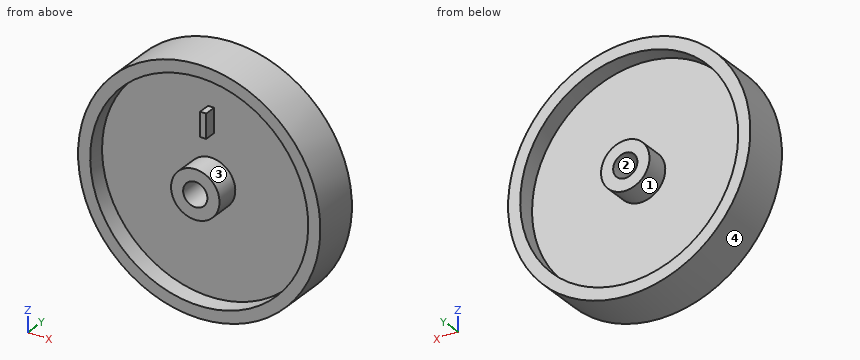
from build123d import *

# Parameters (mm, degrees)
F3_W     = 2.5
F3_H     = 10
F4_DEPTH = 5


with BuildPart() as f2:
    # F0 (on Right) → F2 (revolve)
    with BuildSketch(Plane.YZ):
        Polygon((-25, 5), (0, 5), (0, 10), (-10, 10), (-10, 45), (-2.5, 45), (-2.5, 50), (-22.5, 50), (-22.5, 45), (-15, 45), (-15, 10), (-25, 10), align=None)
    revolve(axis=Axis((0, -23.925491, 0), (0, -1, 0)))

    # F3 (on face) → F4 (join)
    with BuildSketch(Plane.XZ.offset(15)):
        with Locations((0, 25)):
            Rectangle(F3_W, F3_H)
    extrude(amount=F4_DEPTH)


solid = f2.part
Read the model definition and answer for the solid it produces. Units are mm, in the model's axes. Face numbers are marked on the shaded views. A direction names the side the tool comes from. Coordinates: 2 decimals unless noted, no trailing zeros. Write each loop counter-clockwise with the first axis right and the second up, starting at its lowest first coordinate (ties: lowest second). Pieces come first, ordered by that corner, then holes. Notation, with made-up numbers: (-34.5, 22) - (12.5, 22) arc R25 cw to (12.5, 59) - close; hole circle Ø4 at (74.25, 66.5). An arc over 180 degrees is marked (long way). One line per question, with ' | ' between items.
Q1. Find section B-B, the plane x = 0. Write down the section's boundary in (y, z), plus the area to 3 significant figures.
Result set:
outline: (-25, -10) - (-15, -10) - (-15, -45) - (-22.5, -45) - (-22.5, -50) - (-2.5, -50) - (-2.5, -45) - (-10, -45) - (-10, -10) - (0, -10) - (0, -5) - (-25, -5) - close; (-25, 5) - (0, 5) - (0, 10) - (-10, 10) - (-10, 45) - (-2.5, 45) - (-2.5, 50) - (-22.5, 50) - (-22.5, 45) - (-15, 45) - (-15, 30) - (-20, 30) - (-20, 20) - (-15, 20) - (-15, 10) - (-25, 10) - close | area: 850 mm^2
Q2. For the marked faces 1 and 2, determine the directions among +Z, -Z, +X, -X, +Y, -Y from which every point of the face is accessible in a straight line to the end or side of a thin tool.
Result set:
face 1: +Y | face 2: +Y, -Y
Q3. Determine the mould class of the marked faces 3 and 4 for opening direction Z: +Z half, -Z half, draft (parallel to the pull), parting line (faces both ways), or undercut.
Result set:
face 3: undercut | face 4: parting line
Q4. Each of these flat-tipped pins is pushed along its axis until it touches: P1, Ø2.5, axis at y = -18, z = 23.5, coming from the -X side; P2, Ø4, axis at x = 33.5, z = -14.5, coming from the +Y side; P3, Ø2.5, axis at y = -17.5, z = 27, coming from the +X side. Where does it stop, or does it pass through?
Result set:
P1: x = -44.78 | P2: y = -10 | P3: x = 42.86
Q5. Find section C-C, the plane z = 0. Write down the section's boundary in (x, y), plus the area to 3 significant figures.
Result set:
outline: (-50, -22.5) - (-45, -22.5) - (-45, -15) - (-10, -15) - (-10, -25) - (-5, -25) - (-5, 0) - (-10, 0) - (-10, -10) - (-45, -10) - (-45, -2.5) - (-50, -2.5) - close; (5, -25) - (10, -25) - (10, -15) - (45, -15) - (45, -22.5) - (50, -22.5) - (50, -2.5) - (45, -2.5) - (45, -10) - (10, -10) - (10, 0) - (5, 0) - close | area: 800 mm^2
Q6. Consider L1, parallel to Z at x = 0, y = -19; L2, parallel to Z at x = 0, y = -20.25. Determine where each line is inside the solid, lowest interval first. Write a range as [from, to].
Result set:
L1: [-50, -45], [-10, -5], [5, 10], [20, 30], [45, 50] | L2: [-50, -45], [-10, -5], [5, 10], [45, 50]
Q7. Find section A-A, the plane y = -18.5. Write down the section's boundary in (x, z).
Result set:
outline: circle Ø100 at (0, 0); circle Ø20 at (0, 0); (-1.25, 20) - (1.25, 20) - (1.25, 30) - (-1.25, 30) - close; hole circle Ø90 at (0, 0); hole circle Ø10 at (0, 0)
Q8. Find section D-D, the plane z = 23. Write down the section's boundary in (x, y).
Result set:
outline: (-44.4, -22.5) - (-38.68, -22.5) - (-38.68, -15) - (-1.25, -15) - (-1.25, -20) - (1.25, -20) - (1.25, -15) - (38.68, -15) - (38.68, -22.5) - (44.4, -22.5) - (44.4, -2.5) - (38.68, -2.5) - (38.68, -10) - (-38.68, -10) - (-38.68, -2.5) - (-44.4, -2.5) - close
